Read the model definition and answer for the solid it produces. Units are mm, in the model's axes. A direction names the side the tool comes from. Coordinates: 2 decimals unless noted, no trailing zeros. Order: outer loops, then holes, each group sorted by start corner. A loop starts at its lowest first (then second) coordinate and runs counter-clockwise, first axis right, second up. Notation, with made-up numbers: M 18.25,13 L 22.25,13 A20 cw 22.25,45 Z; hole C 46.25,4 d11. An arc over 180 degrees is marked long. One line per question, with ' | ' between items. Start each with the question number.
1) Find section B-B, the plane y = 6. Write down the section's boundary in (x, z) (3 decimals).
2) The mould has two halves that part along Y. Classify faces 1 (the face through (10.427, -19.983, 10.104)), 2 (the face through (0, 8.725, 7)), 3 (the face through (-11.215, -19, 10)), 4 (the face through (17.194, -0.078, 6.434)): +Y half, -Y half, draft (parallel to the pull), parting line (faces both ways), or undercut.
3) Find section A-A, the plane x = 0. Write down the section's boundary in (y, z) (3 decimals).
4) Find section C-C, the plane x = 6. Write down the section's boundary in (y, z) (3 decimals), plus the area to 3 significant figures.
5) Find section D-D, the plane y = 1. Write down the section's boundary in (x, z).
6) Consider probe 1 along X at (y, z) = (5, 2.25) (3 decimals); probe 2 along X at (y, z) = (-17.5, 4.75) (3 decimals); probe 3 along Z at (x, y) = (4.5, 10.5). Determine where each line is inside the solid, lowest interval first.
7) Given P1, Ø3, axis at y = 6.5, z = 4, coming from the -X side (3 decimals); P2, Ø7, axis at y = -6, z = 8, coming from the +X side; P3, Ø2, axis at y = 11, z = 2, coming from the +X side (3 decimals); P4, Ø1.5, axis at x = 9.5, y = -11.5, coming from the -Z side, each flat-ended and moving along its own axis, determine where each tip first touches the part or whether it passes through.
8) A tool of negligible diameter and unlimited length cuts with its end or side. For faces 5 (the face through (9.515, -19, 10)), 6 (the face through (10.115, -10, 6)), 7 (the face through (-12, -3.54, 6)), 8 (the face through (-16.194, 0.056, 6.863)), from which of +Z, -Z, +X, -X, +Y, -Y can it reach the whole face along a straight path? Write none if from no direction.
from build123d import *

# Parameters (mm, degrees)
F0_W      = 20.23
F0_H      = 6.185
F1_DEPTH  = 13.05
F2_W      = 18.23
F2_H      = 17.45
F3_DEPTH  = 12.55
F5_DEPTH  = 12.55
F6_R      = 7.95
F7_DEPTH  = 0.501
F8_W      = 20.23
F8_H      = 13.05
F9_DEPTH  = 10
F10_W     = 20.23
F10_H     = 9.9667743579
F11_DEPTH = 25
F13_DEPTH = 27.311
F15_DEPTH = 27.311
F17_W     = 20.23
F17_H     = 13.05
F18_DEPTH = 8.2
F20_DEPTH = 25
F22_DEPTH = 2
F23_DEPTH = 2
F25_DEPTH = 29.311
F27_DEPTH = 1.65


with BuildPart() as f1:
    # F0 (on Top) → F1 (new body)
    with BuildSketch(Plane.XY):
        with Locations((0, -6.6325)):
            Rectangle(F0_W, F0_H)
        Polygon((-10.115, -3.54), (10.115, -3.54), (10.115, 0), (10.115, 3.54), (-10.115, 3.54), (-10.115, 0), align=None)
        with BuildLine():
            Line((10.115, 0), (10.115, -3.54))
            Line((10.115, -3.54), (13.655, -3.54))
            ThreePointArc((13.655, -3.54), (11.1518419946, -2.5031580054), (10.115, 0))
        make_face()
        with BuildLine():
            Line((-13.655, -3.54), (-10.115, -3.54))
            Line((-10.115, -3.54), (-10.115, 0))
            ThreePointArc((-10.115, 0), (-11.1518419946, -2.5031580054), (-13.655, -3.54))
        make_face()
        with BuildLine():
            Line((10.115, 3.54), (10.115, 0))
            ThreePointArc((10.115, 0), (11.1518419946, 2.5031580054), (13.655, 3.54))
            Line((13.655, 3.54), (10.115, 3.54))
        make_face()
        with BuildLine():
            ThreePointArc((13.655, 3.54), (11.1518419946, 2.5031580054), (10.115, 0))
            ThreePointArc((10.115, 0), (11.1518419946, -2.5031580054), (13.655, -3.54))
            Line((13.655, -3.54), (13.655, 3.54))
        make_face()
        with BuildLine():
            Line((13.655, 3.54), (13.655, -3.54))
            ThreePointArc((13.655, -3.54), (16.1581580054, -2.5031580054), (17.195, 0))
            ThreePointArc((17.195, 0), (16.1581580054, 2.5031580054), (13.655, 3.54))
        make_face()
        with BuildLine():
            ThreePointArc((-13.655, 3.54), (-11.1518419946, 2.5031580054), (-10.115, 0))
            Line((-10.115, 0), (-10.115, 3.54))
            Line((-10.115, 3.54), (-13.655, 3.54))
        make_face()
        with BuildLine():
            ThreePointArc((-13.655, -3.54), (-11.1518419946, -2.5031580054), (-10.115, 0))
            ThreePointArc((-10.115, 0), (-11.1518419946, 2.5031580054), (-13.655, 3.54))
            Line((-13.655, 3.54), (-13.655, -3.54))
        make_face()
        with BuildLine():
            ThreePointArc((-13.655, 3.54), (-17.195, 0), (-13.655, -3.54))
            Line((-13.655, -3.54), (-13.655, 3.54))
        make_face()
        with Locations((0, 6.6325)):
            Rectangle(F0_W, F0_H)
    extrude(amount=F1_DEPTH)

    # F2 (on face) → F3 (cut)
    with BuildSketch(Plane.XY.offset(13.05)):
        Rectangle(F2_W, F2_H)
    extrude(amount=-F3_DEPTH, mode=Mode.SUBTRACT)

    # F4 (on face) → F5 (cut)
    with BuildSketch(Plane.XY.offset(13.05)):
        with BuildLine():
            ThreePointArc((-13.655, -2.54), (-11.8589487758, -1.7960512242), (-11.115, 0))
            ThreePointArc((-11.115, 0), (-11.8589487758, 1.7960512242), (-13.655, 2.54))
            Line((-13.655, 2.54), (-13.655, -2.54))
        make_face()
        with BuildLine():
            ThreePointArc((-13.655, 2.54), (-11.8589487758, 1.7960512242), (-11.115, 0))
            ThreePointArc((-11.115, 0), (-11.8589487758, -1.7960512242), (-13.655, -2.54))
            Line((-13.655, -2.54), (13.655, -2.54))
            ThreePointArc((13.655, -2.54), (11.115, 0), (13.655, 2.54))
            Line((13.655, 2.54), (-13.655, 2.54))
        make_face()
        with BuildLine():
            Line((-13.655, -2.54), (-13.655, 2.54))
            ThreePointArc((-13.655, 2.54), (-16.195, 0), (-13.655, -2.54))
        make_face()
        with BuildLine():
            Line((13.655, -2.54), (13.655, 2.54))
            ThreePointArc((13.655, 2.54), (11.115, 0), (13.655, -2.54))
        make_face()
        with BuildLine():
            ThreePointArc((16.195, 0), (15.4510512242, 1.7960512242), (13.655, 2.54))
            Line((13.655, 2.54), (13.655, -2.54))
            ThreePointArc((13.655, -2.54), (15.4510512242, -1.7960512242), (16.195, 0))
        make_face()
    extrude(amount=-F5_DEPTH, mode=Mode.SUBTRACT)

    # F6 (on face) → F7 (cut, through all)
    with BuildSketch(Plane.XY.offset(0.5)):
        Circle(F6_R)
    extrude(amount=-F7_DEPTH, mode=Mode.SUBTRACT)

    # F8 (on face) → F9 (join)
    with BuildSketch(Plane.XZ.offset(9.725)):
        with Locations((0, 6.525)):
            Rectangle(F8_W, F8_H)
    extrude(amount=F9_DEPTH)

    # F10 (on face) → F11 (join)
    with BuildSketch(Plane.XY.offset(13.05)):
        with Locations((0, -14.7416128211)):
            Rectangle(F10_W, F10_H)
    extrude(amount=F11_DEPTH)

    # F12 (on face) → F13 (cut, through all)
    with BuildSketch(Plane(origin=(-10.115, 0, 0), x_dir=(0, -1, 0), z_dir=(-1, 0, 0))):
        Polygon((19.725, 38.05), (14.4232781604, 38.05), (19.725, 0), align=None)
    extrude(amount=-F13_DEPTH, mode=Mode.SUBTRACT)

    # F14 (on face) → F15 (cut, through all)
    with BuildSketch(Plane(origin=(-10.115, 0, 0), x_dir=(0, -1, 0), z_dir=(-1, 0, 0))):
        Polygon((9.7582256421, 13.05), (14.8776879954, 13.05), (11.4232781604, 38.05), (9.7582256421, 38.05), align=None)
    extrude(amount=-F15_DEPTH, mode=Mode.SUBTRACT)

    # F17 (on face) → F18 (join)
    with BuildSketch(Plane(origin=(0, 9.725, 0), x_dir=(-1, 0, 0), z_dir=(0, 1, 0))):
        with Locations((0, 6.525)):
            Rectangle(F17_W, F17_H)
    extrude(amount=F18_DEPTH)

    # F19 (on face) → F20 (cut)
    with BuildSketch(Plane.YZ.offset(10.115)):
        Polygon((17.925, 0), (17.925, 13.05), (16.1217980661, 0), align=None)
    extrude(amount=-F20_DEPTH, mode=Mode.SUBTRACT)

    # F21 (on face) → F22 (join)
    with BuildSketch(Plane(origin=(-10.115, 0, 0), x_dir=(0, -1, 0), z_dir=(-1, 0, 0))):
        Polygon((19.725, 0), (14.4232781604, 38.05), (11.4232781604, 38.05), (16.6808899293, 0), align=None)
    extrude(amount=F22_DEPTH)

    # F16 (on face) → F23 (join)
    with BuildSketch(Plane.YZ.offset(10.115)):
        Polygon((-11.4232781604, 38.05), (-14.4232781604, 38.05), (-19.725, 0), (-16.6808899293, 0), (-14.8776879954, 13.05), align=None)
    extrude(amount=F23_DEPTH)

    # F24 (on face) → F25 (cut, through all)
    with BuildSketch(Plane(origin=(-12.115, 0, 0), x_dir=(0, -1, 0), z_dir=(-1, 0, 0))):
        Polygon((11.4232781604, 38.05), (13.9726326186, 19.6), (16.9940210761, 19.6), (14.4232781604, 38.05), align=None)
    extrude(amount=-F25_DEPTH, mode=Mode.SUBTRACT)

    # F26 (on face) → F27 (join)
    with BuildSketch(Plane(origin=(0, -19.349343601, 2.6960535493), x_dir=(1, 0, 0), z_dir=(0, -0.9904318834, 0.1380024795))):
        with BuildLine():
            ThreePointArc((-11.215, 13.1029010909), (-10.29, 12.1779010909), (-9.365, 13.1029010909))
            ThreePointArc((-9.365, 13.1029010909), (-10.29, 14.0279010909), (-11.215, 13.1029010909))
        make_face()
        with BuildLine():
            Line((-9.365, 1.2029010909), (-9.365, 13.1029010909))
            ThreePointArc((-9.365, 13.1029010909), (-10.29, 12.1779010909), (-11.215, 13.1029010909))
            Line((-11.215, 13.1029010909), (-11.215, 1.2029010909))
            ThreePointArc((-11.215, 1.2029010909), (-10.29, 2.1279010909), (-9.365, 1.2029010909))
        make_face()
        with BuildLine():
            ThreePointArc((-11.215, 1.2029010909), (-10.29, 0.2779010909), (-9.365, 1.2029010909))
            ThreePointArc((-9.365, 1.2029010909), (-10.29, 2.1279010909), (-11.215, 1.2029010909))
        make_face()
        with BuildLine():
            ThreePointArc((9.515, 13.1029010909), (10.44, 12.1779010909), (11.365, 13.1029010909))
            ThreePointArc((11.365, 13.1029010909), (10.44, 14.0279010909), (9.515, 13.1029010909))
        make_face()
        with BuildLine():
            Line((11.365, 1.2029010909), (11.365, 13.1029010909))
            ThreePointArc((11.365, 13.1029010909), (10.44, 12.1779010909), (9.515, 13.1029010909))
            Line((9.515, 13.1029010909), (9.515, 1.2029010909))
            ThreePointArc((9.515, 1.2029010909), (10.44, 2.1279010909), (11.365, 1.2029010909))
        make_face()
        with BuildLine():
            ThreePointArc((9.515, 1.2029010909), (10.44, 0.2779010909), (11.365, 1.2029010909))
            ThreePointArc((11.365, 1.2029010909), (10.44, 2.1279010909), (9.515, 1.2029010909))
        make_face()
    extrude(amount=F27_DEPTH)


solid = f1.part
Report:
1) outline: M -10.115,0 L -5.216,0 L -5.216,0.5 L -9.115,0.5 L -9.115,13.05 L -10.115,13.05 Z; M 5.216,0 L 10.115,0 L 10.115,13.05 L 9.115,13.05 L 9.115,0.5 L 5.216,0.5 Z
2) face 1: -Y half | face 2: undercut | face 3: draft | face 4: parting line
3) outline: M -19.725,0 L -7.95,0 L -7.95,0.5 L -8.725,0.5 L -8.725,13.05 L -14.878,13.05 L -13.973,19.6 L -16.994,19.6 Z; M 7.95,0 L 16.122,0 L 17.925,13.05 L 8.725,13.05 L 8.725,0.5 L 7.95,0.5 Z
4) outline: M -19.725,0 L -5.216,0 L -5.216,0.5 L -8.725,0.5 L -8.725,13.05 L -14.878,13.05 L -13.973,19.6 L -16.994,19.6 Z; M 5.216,0 L 16.122,0 L 17.925,13.05 L 8.725,13.05 L 8.725,0.5 L 5.216,0.5 Z | area: 263 mm^2
5) outline: M -17.05,0 L -7.89,0 L -7.89,0.5 L -15.99,0.5 L -15.99,13.05 L -17.05,13.05 Z; M 7.89,0 L 17.05,0 L 17.05,13.05 L 15.99,13.05 L 15.99,0.5 L 7.89,0.5 Z
6) probe 1: x = -10.115 to -9.115, 9.115 to 10.115 | probe 2: x = -12.115 to 12.115 | probe 3: z = 0 to 13.05
7) P1: stops at x = -10.115 | P2: stops at x = 16.16 | P3: stops at x = 10.115 | P4: stops at z = 0
8) face 5: +Z, -Y | face 6: -Z, +X | face 7: +Z, -Z, -X | face 8: +Z
